from build123d import *

# Parameters (mm, degrees)
SKETCH_1_W          = 9.29
SKETCH_1_H          = 1.5
REVOLVE_1_ANGLE     = 180
EXTRUDE_1_DEPTH     = 4.65
SKETCH_3_W          = 18.62
SKETCH_3_H          = 6.156693915
EXTRUDE_2_DEPTH     = 15.87
FILLET_1_R          = 1
CUT_EXTRUDE_1_DEPTH = 0.01


with BuildPart() as part:
    # 草图1 → 旋转1 (revolve)
    with BuildSketch(Plane.XZ):
        with Locations((-4.646272468, 0.75)):
            Rectangle(SKETCH_1_W, SKETCH_1_H)
    revolve(axis=Axis((-0.001272468, 0, 0), (0, 0, -1)), revolution_arc=REVOLVE_1_ANGLE)

    # 草图2 → 凸台-拉伸1 (add)
    with BuildSketch(Plane.XY.offset(1.5)):
        with BuildLine():
            Line((-9.291272468, 0), (9.288727532, 0))
            ThreePointArc((9.288727532, 0), (-0.001272468, 9.29), (-9.291272468, 0))
        make_face()
    extrude(amount=EXTRUDE_1_DEPTH)

    # 草图3 → 凸台-拉伸2 (add)
    with BuildSketch(Plane.XZ):
        with Locations((-0.001272468, 3.078346957)):
            Rectangle(SKETCH_3_W, SKETCH_3_H)
    extrude(amount=EXTRUDE_2_DEPTH)

    # 圆角1
    fillet_1_edges = [part.edges().sort_by_distance(p)[0] for p in [
        (9.308727532, -15.87, 3.078346957),
        (-9.311272468, -15.87, 3.078346957),
    ]]
    fillet(fillet_1_edges, radius=FILLET_1_R)

    # 草图4 → 切除-拉伸1 (cut)
    with BuildSketch(Plane.XY.offset(6.15)):
        with BuildLine():
            Line((-9.291272468, 0), (9.288727532, 0))
            ThreePointArc((9.288727532, 0), (-0.001272468, 9.29), (-9.291272468, 0))
        make_face()
    extrude(amount=-CUT_EXTRUDE_1_DEPTH, mode=Mode.SUBTRACT)


solid = part.part
Geometry: final body of the model. Coordinates: model frame, mm. Give positions to 0.01 mm unless a question says otherwise; leave off trailing zeros. Write each loop counter-clockwise with the first axis right and the second up, starting at its lowest first coordinate (ties: lowest second). Pieces come first, ordered by that corner, then holes. Notation, with made-up numbers: (88.25, 47) -> (105.25, 47) arc R16 cw to (105.25, 58) -> close; hole circle Ø10 at (-36, 45.5). An arc over 180 degrees is marked (long way). Answer as a JSON object with one key per item and string values.
1. Contact query for flat-ended pins moving along their axis: pin 1 (7.5 mm diameter, centred on x = 4.5, y = 5.5, fed in from +Z); pin 2 (1 mm diameter, centred on x = -2, z = 1, fed in from +Y). Output: stop coordinate, or through.
Ans:
{"pin 1": "stops at z = 6.14", "pin 2": "stops at y = 9.17"}
2. Ray query, probe 1 along Z at (x, y) = (-4.25, 6.75); probe 2 along X at (y, z) = (0.25, 3.5); probe 3 along Y at (x, z) = (2.75, 5.5). Return the intervals inside material, ascending. Write a range as from..to.
Ans:
{"probe 1": "z = 0..6.14", "probe 2": "x = -9.29..9.29", "probe 3": "y = -15.87..8.87"}
3. Cut plane C-C on y = 3.5. Output: boundary loops of the cut face in (x, z), and give its area (3 significant figures).
Ans:
{"outline": "(-8.61, 0) -> (8.6, 0) -> (8.6, 6.14) -> (-8.61, 6.14) -> close", "area": "106 mm^2"}
